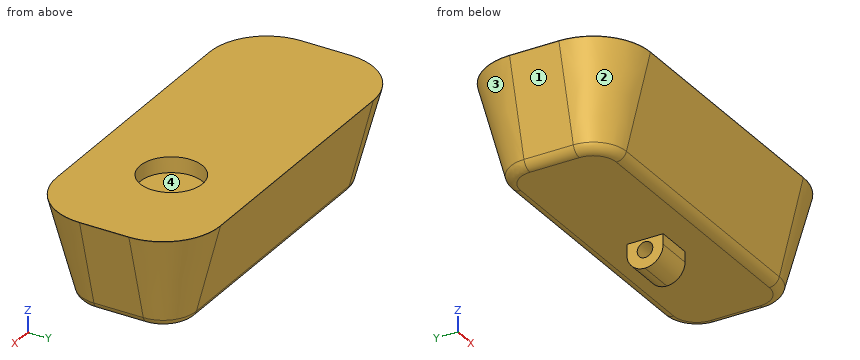
```python
from build123d import *

# Parameters (mm, degrees)
SKETCH1_W           = 71
SKETCH1_H           = 31.5
BOSS_EXTRUDE1_DEPTH = 9.5
FILLET1_R           = 11
CHAMFER1_SIZE       = 5
CHAMFER1_SIZE2      = 18.924240442
SKETCH2_W           = 5.5
SKETCH2_H           = 7
BOSS_EXTRUDE2_DEPTH = 7
FILLET2_R           = 3.5
SKETCH3_R           = 1.5
CUT_EXTRUDE1_DEPTH  = 7
FILLET3_R           = 2
SKETCH4_R           = 6
CUT_EXTRUDE2_DEPTH  = 3


with BuildPart() as part:
    # Sketch1 → Boss-Extrude1 (new, symmetric)
    with BuildSketch(Plane.XY):
        Rectangle(SKETCH1_W, SKETCH1_H)
    extrude(amount=BOSS_EXTRUDE1_DEPTH, both=True)

    # Fillet1
    fillet1_edges = [part.edges().sort_by_distance(p)[0] for p in [
        (-35.5, 15.75, 0),
        (35.5, 15.75, 0),
        (35.5, -15.75, 0),
        (-35.5, -15.75, 0),
    ]]
    fillet(fillet1_edges, radius=FILLET1_R)

    # Chamfer1
    chamfer1_edges = [part.edges().sort_by_distance(p)[0] for p in [
        (0, -15.75, -9.5),
        (-35.5, 0, -9.5),
        (0, 15.75, -9.5),
        (35.5, 0, -9.5),
        (32.278174593, 12.528174593, -9.5),
        (32.278174593, -12.528174593, -9.5),
        (-32.278174593, 12.528174593, -9.5),
        (-32.278174593, -12.528174593, -9.5),
    ]]
    chamfer1_side = [part.faces().sort_by_distance(p)[0] for p in [
        (0, 0, -9.5),
    ]]
    chamfer(chamfer1_edges, length=CHAMFER1_SIZE, length2=CHAMFER1_SIZE2, reference=chamfer1_side[0])

    # Sketch2 → Boss-Extrude2 (add)
    with BuildSketch(Plane(origin=(0, 0, 0), x_dir=(0, 0, -1), z_dir=(1, 0, 0))):
        with Locations((12.25, 0)):
            Rectangle(SKETCH2_W, SKETCH2_H)
    extrude(amount=BOSS_EXTRUDE2_DEPTH)

    # Fillet2
    fillet2_edges = [part.edges().sort_by_distance(p)[0] for p in [
        (3.5, -3.5, -15),
        (3.5, 3.5, -15),
    ]]
    fillet(fillet2_edges, radius=FILLET2_R - 0.0001)  # a hair under: the kernel refuses the full size

    # Sketch3 → Cut-Extrude1 (cut)
    with BuildSketch(Plane(origin=(7, 0, 0), x_dir=(0, 0, -1), z_dir=(1, 0, 0))):
        with Locations((11.5, 0)):
            Circle(SKETCH3_R)
    extrude(amount=-CUT_EXTRUDE1_DEPTH, mode=Mode.SUBTRACT)

    # Fillet3
    fillet3_edges = [part.edges().sort_by_distance(p)[0] for p in [
        (0, 10.75, -9.5),
        (-28.742640687, 8.992640687, -9.5),
        (28.742640687, 8.992640687, -9.5),
        (-30.5, 0, -9.5),
        (30.5, 0, -9.5),
        (-28.742640687, -8.992640687, -9.5),
        (28.742640687, -8.992640687, -9.5),
        (0, -10.75, -9.5),
    ]]
    fillet(fillet3_edges, radius=FILLET3_R)

    # Sketch4 → Cut-Extrude2 (cut)
    with BuildSketch(Plane.XY.offset(9.5)):
        with Locations((14, 0)):
            Circle(SKETCH4_R)
    extrude(amount=-CUT_EXTRUDE2_DEPTH, mode=Mode.SUBTRACT)


solid = part.part
```
Design review of the part built by this model. Coordinates are the model's own, in mm. Face numbers are marked on the shaded views. Give positions to 0.01 mm unless a question says otherwise; leave off trailing zeros. Loops run counter-clockwise (first coordinate to the right, second up) from the corner with the lowest first, then second, coordinate; pieces in that order, holes last. Notation, with made-up numbers: (-20.5, 54) -> (20.5, 54) arc R23 ccw to (20.5, 72) -> close; hole circle Ø7 at (-20.5, 28). An arc over 180 degrees is marked (long way). One line per item, written item: value.
Q1. For L1, parallel to Z at x = 0.5, y = 7; L2, parallel to Z at x = 11.5, y = -2.5; L3, parallel to Y at x = 14, z = 7.2, list the stretches that pass through material, from the lowest coordinate up.
Numbers:
L1: z = -9.5 to 9.5
L2: z = -9.5 to 6.5
L3: y = -15.16 to -6, 6 to 15.16
Q2. For pin 1 Ø6 at (x, z) = (0.5, -9) entering from -Y; pin 2 Ø5 at (x, z) = (14, 3) entering from -Y; pin 3 Ø0.6 at (x, z) = (5, -10) entering from -Y, all flat-tipped, find the tip position at first contact; note any pin that passes through.
Numbers:
pin 1: stops at y = -11.67
pin 2: stops at y = -14.71
pin 3: stops at y = -3.5
Q3. We need section D-D on x = 14. Give the boundary of the cut face in (y, z), and give its area (3 significant figures).
Numbers:
outline: (-15.75, 9.42) -> (-11.14, -8.01) arc R2 ccw to (-9.21, -9.5) -> (9.21, -9.5) arc R2 ccw to (11.14, -8.01) -> (15.75, 9.42) -> (15.75, 9.5) -> (6, 9.5) -> (6, 6.5) -> (-6, 6.5) -> (-6, 9.5) -> (-15.75, 9.5) -> close
area: 467 mm^2
Q4. We need section B-B on z = 7.25. Give the boundary of the cut face in (x, y), and give its area (3 significant figures).
Numbers:
outline: (-34.93, -4.75) arc R10.43 ccw to (-24.5, -15.18) -> (24.5, -15.18) arc R10.43 ccw to (34.93, -4.75) -> (34.93, 4.75) arc R10.43 ccw to (24.5, 15.18) -> (-24.5, 15.18) arc R10.43 ccw to (-34.93, 4.75) -> close; hole circle Ø12 at (14, 0)
area: 1,910 mm^2
Q5. Draft analysis for pull direction Y (two halves, no side actions). For the marked faces 1, 2, 3 and 4, state which applies: pulls with the +Y half, pulls with the -Y half, needs draft (parallel to the pull), parting line crosses it, or undercut.
Numbers:
face 1: needs draft
face 2: pulls with the -Y half
face 3: pulls with the +Y half
face 4: undercut
Q6. We need section A-A on x = -6. Give the boundary of the cut face in (y, z), and give its area (3 significant figures).
Numbers:
outline: (-15.75, 9.42) -> (-11.14, -8.01) arc R2 ccw to (-9.21, -9.5) -> (9.21, -9.5) arc R2 ccw to (11.14, -8.01) -> (15.75, 9.42) -> (15.75, 9.5) -> (-15.75, 9.5) -> close
area: 503 mm^2
Q7. We need section C-C on z = -1.5. Give the boundary of the cut face in (x, y).
Numbers:
outline: (-32.61, -4.75) arc R8.11 ccw to (-24.5, -12.86) -> (24.5, -12.86) arc R8.11 ccw to (32.61, -4.75) -> (32.61, 4.75) arc R8.11 ccw to (24.5, 12.86) -> (-24.5, 12.86) arc R8.11 ccw to (-32.61, 4.75) -> close
